from build123d import *

# Parameters (mm, degrees)
SKETCH_1_R          = 18
SKETCH_1_R_2        = 15
EXTRUDE_1_DEPTH     = 20
SKETCH_2_R          = 18
EXTRUDE_2_DEPTH     = 3
SKETCH_3_R          = 7.5
SKETCH_3_R_2        = 4.5
EXTRUDE_3_DEPTH     = 20
CUT_EXTRUDE_START   = -20
SKETCH_4_R          = 4.5
CUT_EXTRUDE_1_DEPTH = 20
SKETCH_5_R          = 7.5
EXTRUDE_4_DEPTH     = 5
SKETCH_6_R          = 4
EXTRUDE_5_DEPTH     = 20
SKETCH_7_R          = 1.75
CUT_EXTRUDE_2_DEPTH = 15
FILLET_1_R          = 2
FILLET_2_R          = 1.5


with BuildPart() as part:
    # 草图1 → 凸台-拉伸1 (new body)
    with BuildSketch(Plane.XY):
        Circle(SKETCH_1_R)
        Circle(SKETCH_1_R_2, mode=Mode.SUBTRACT)
    extrude(amount=EXTRUDE_1_DEPTH)

    # 草图2 → 凸台-拉伸2 (add)
    with BuildSketch(Plane.XY.offset(20)):
        Circle(SKETCH_2_R)
    extrude(amount=EXTRUDE_2_DEPTH)

    # 草图3 → 凸台-拉伸3 (add)
    with BuildSketch(Plane.XY.offset(23)):
        Circle(SKETCH_3_R)
        Circle(SKETCH_3_R_2, mode=Mode.SUBTRACT)
    extrude(amount=EXTRUDE_3_DEPTH)

    # 草图4 → 切除-拉伸1 (cut)
    with BuildSketch(Plane.XY.offset(23).offset(CUT_EXTRUDE_START)):
        Circle(SKETCH_4_R)
    extrude(amount=CUT_EXTRUDE_1_DEPTH, mode=Mode.SUBTRACT)

    # 草图5 → 凸台-拉伸4 (add)
    with BuildSketch(Plane.XY.offset(43)):
        Circle(SKETCH_5_R)
    extrude(amount=EXTRUDE_4_DEPTH)

    # 草图6 → 凸台-拉伸5 (add)
    with BuildSketch(Plane.XY.offset(48)):
        Circle(SKETCH_6_R)
    extrude(amount=EXTRUDE_5_DEPTH)

    # 草图7 → 切除-拉伸2 (cut)
    with BuildSketch(Plane.XY.offset(23)):
        with Locations((0, 12.5)):
            Circle(SKETCH_7_R)
        with Locations((12.5, 0)):
            Circle(SKETCH_7_R)
        with Locations((0, -12.5)):
            Circle(SKETCH_7_R)
        with Locations((-12.5, 0)):
            Circle(SKETCH_7_R)
    extrude(amount=-CUT_EXTRUDE_2_DEPTH, mode=Mode.SUBTRACT)

    # 圆角1
    fillet_1_edges = [part.edges().sort_by_distance(p)[0] for p in [
        (-4, 0, 48),
    ]]
    fillet(fillet_1_edges, radius=FILLET_1_R)

    # 圆角2
    fillet_2_edges = [part.edges().sort_by_distance(p)[0] for p in [
        (-7.5, 0, 23),
    ]]
    fillet(fillet_2_edges, radius=FILLET_2_R)


solid = part.part
The model under review builds one solid part; all positions refer to its coordinate system, in mm. A direction names the side the tool comes from. Give positions to 0.01 mm unless a question says otherwise; leave off trailing zeros. Loops run counter-clockwise (first coordinate to the right, second up) from the corner with the lowest first, then second, coordinate; pieces in that order, holes last. Notation, with made-up numbers: (47, 28.25) -> (99, 28.25) arc R22 cw to (99, 54.25) -> close; hole circle Ø9 at (73.5, 12.5). An arc over 180 degrees is marked (long way). Answer as a JSON object with one key per item and string values. Group by question number.
Q1. Draft analysis for pull direction Y (two halves, no side actions). For faces 4 (the flat face through (3, 4, 20)), 5 (the cylindrical face through (-0.228, -10.765, 21.521)), 6 (the cylindrical face through (-0.867, -3.905, 58.874)), 7 (the flat face through (-8.3, 4.3, 23)), state which applies: pulls with the +Y half, pulls with the -Y half, needs draft (parallel to the pull), parting line crosses it, or undercut.
Q2. Wall thickness on line 1 along Y through (x, z) = (0, 21.25); line 2 along Y through (x, z) = (0, 37.5); line 3 along Z through (x, y) = (-12.5, 3.5): over which ranges is each line inside the solid? List them lowest first.
Q3. Take a section at C-C (y = -12.5). Write out the cut boundary in (x, z).
Q4. Take a section at A-A (x = 0). State how many separate pieces and enclosed holes the cut face has, plus the area to 3 significant figures.
Q5. Tool access review of faces 1 (the cylindrical face through (-0.59, 4.46, 31.34)), 2 (the cylindrical face through (-0.228, 14.235, 21.521)), 3 (the cylindrical face through (-7.493, 0.33, 36.085)): name each direction out of +Z, -Z, +X, -X, +Y, -Y from which nothing blocks a thin tool from reaching the whole face with its end or side.
Q6. Insertion check: pin 1 (1 mm diameter, centred on y = 3.5, z = 39.5, fed in from -X); pin 2 (4 mm diameter, centred on y = 7, z = 33.5, fed in from +X); pin 3 (2 mm diameter, centred on x = 0, y = -12.5, fed in from -Z); pin 4 (1.5 mm diameter, centred on x = -7, z = 25, fed in from -Y). Each pin has a flat end and moves straight along its axis. Give the tip position at first contact, or say it passes through.
Answer below:
{
 "1": {"face 4": "undercut", "face 5": "undercut", "face 6": "parting line crosses it", "face 7": "needs draft"},
 "2": {"line 1": "y = -18 to -14.25, -10.75 to -4.5, 4.5 to 10.75, 14.25 to 18", "line 2": "y = -7.5 to -4.5, 4.5 to 7.5", "line 3": "z = 20 to 23"},
 "3": {"outline": "(-12.95, 0) -> (-8.29, 0) -> (-8.29, 20) -> (-1.75, 20) -> (-1.75, 23) -> (-12.95, 23) -> close; (1.75, 20) -> (8.29, 20) -> (8.29, 0) -> (12.95, 0) -> (12.95, 23) -> (1.75, 23) -> close"},
 "4": {"separate pieces": "3", "enclosed holes": "0", "area": "538 mm2"},
 "5": {"face 1": "-Z", "face 2": "+Z, -Z", "face 3": "+Z"},
 "6": {"pin 1": "stops at x = -6.87", "pin 2": "stops at x = 5.59", "pin 3": "passes through", "pin 4": "stops at y = -4.15"}
}
